Autodesk Inventor part; units mm, degrees
ref_plane "YZ Plane" through (0, 0, 0) normal (1, 0, 0) x (0, 1, 0)
ref_plane "XZ Plane" through (0, 0, 0) normal (0, 1, 0) x (-1, 0, 0)
ref_plane "XY Plane" through (0, 0, 0) normal (0, 0, 1) x (1, 0, 0)
sketch "Sketch1" plane through (0, 0, 0) normal (0, 0, 1) x (1, 0, 0)
  line L0 (0, 0) -> (850.9, 0)
  line L1 (850.9, 0) -> (850.9, 76.2)
  line L2 (850.9, 76.2) -> (0, 76.2)
  line L3 (0, 76.2) -> (0, 0)
  dimension "d0" = 850.9
  dimension "d1" = 76.2
extrude "Extrusion1" add sketch "Sketch1" along normal blind 3.175
sketch "Sketch4" plane through (0, 0, 3.175) normal (0, 0, 1) x (1, 0, 0)
  line L0 (0, 0) -> (0, 38.1)
  line L1 (0, 76.2) -> (0, 0)
  line L2 (0, 0) -> (25.4, 0)
  line L3 (0, 0) -> (850.9, 0)
  line L4 (25.4, 0) -> (0, 38.1)
  line L5 (850.9, 0) -> (825.5, 0)
  line L6 (850.9, 0) -> (850.9, 38.1)
  line L7 (850.9, 0) -> (850.9, 76.2)
  line L8 (850.9, 38.1) -> (825.5, 0)
  line L9 (0, 38.1) -> (0, 36.5125)
  circle A0 centre (292.9509, 36.5125) radius 14.2875
  circle A1 centre (557.9491, 36.5125) radius 14.2875
  circle A2 centre (757.9743, 39.6875) radius 14.2875
  circle A3 centre (92.9257, 39.6875) radius 14.2875
  dimension "d24" = 38.1
  dimension "d26" = 25.4
  dimension "d27" = 38.1
  dimension "d33" = 28.575
  dimension "d34" = 28.575
  dimension "d38" = 28.575
  dimension "d39" = 28.575
extrude "Extrusion3" cut sketch "Sketch4" against normal blind 3.175
sketch "Sketch5" plane through (0, 0, 3.175) normal (0, 0, 1) x (1, 0, 0)
  line L0 (850.9, 76.2) -> (0, 76.2)
  line L1 (0, 76.2) -> (425.45, 76.2)
  circle A0 centre (425.45, 66.675) radius 3.5687
  circle A1 centre (425.45, 9.525) radius 3.5687
  line L2 (25.4, 0) -> (825.5, 0)
  line L3 (0, 76.2) -> (190.5, 76.2)
  circle A2 centre (190.5, 66.675) radius 3.5687
  circle A3 centre (190.5, 9.525) radius 3.5687
  circle A4 centre (190.5, 38.1) radius 3.5687
  line L4 (850.9, 38.1) -> (850.9, 76.2)
  line L5 (850.9, 76.2) -> (660.4, 76.2)
  circle A5 centre (660.4, 66.675) radius 3.5687
  circle A6 centre (660.4, 9.525) radius 3.5687
  circle A7 centre (660.4, 38.1) radius 3.5687
  circle A8 centre (838.2, 63.5) radius 3.5687
  circle A9 centre (12.7, 63.5) radius 3.5687
  line L6 (0, 76.2) -> (0, 38.1)
  circle A10 centre (34.925, 12.7) radius 3.5687
  circle A11 centre (815.975, 12.7) radius 3.5687
  point P0 (0, 0)
  dimension "d42" = 425.45
  dimension "d43" = 7.1374
  dimension "d44" = 9.525
  dimension "d45" = 7.1374
  dimension "d46" = 9.525
  dimension "d47" = 190.5
  dimension "d48" = 7.1374
  dimension "d49" = 9.525
  dimension "d50" = 7.1374
  dimension "d51" = 9.525
  dimension "d52" = 7.1374
  dimension "d53" = 38.1
  dimension "d54" = 190.5
  dimension "d55" = 7.1374
  dimension "d56" = 9.525
  dimension "d57" = 7.1374
  dimension "d58" = 9.525
  dimension "d59" = 7.1374
  dimension "d60" = 38.1
  dimension "d61" = 7.1374
  dimension "d62" = 12.7
  dimension "d63" = 12.7
  dimension "d64" = 7.1374
  dimension "d65" = 12.7
  dimension "d66" = 12.7
  dimension "d67" = 7.1374
  dimension "d69" = 12.7
  dimension "d70" = 9.525
  dimension "d71" = 7.1374
  dimension "d72" = 12.7
  dimension "d73" = 9.525
extrude "Extrusion4" cut sketch "Sketch5" against normal blind 3.175
sketch "Sketch6" plane through (0, 0, 3.175) normal (0, 0, 1) x (1, 0, 0)
  circle A0 centre (190.5, 38.1) radius 3.5687
  circle A1 centre (660.4, 38.1) radius 3.5687
  line L0 (177.673, 25.273) -> (203.327, 25.273)
  line L1 (203.327, 25.273) -> (203.327, 50.927)
  line L2 (203.327, 50.927) -> (177.673, 50.927)
  line L3 (177.673, 50.927) -> (177.673, 25.273)
  line L4 (177.673, 25.273) -> (203.327, 50.927) construction
  line L5 (203.327, 25.273) -> (177.673, 50.927) construction
  line L6 (647.573, 25.273) -> (673.227, 25.273)
  line L7 (673.227, 25.273) -> (673.227, 50.927)
  line L8 (673.227, 50.927) -> (647.573, 50.927)
  line L9 (647.573, 50.927) -> (647.573, 25.273)
  line L10 (647.573, 25.273) -> (673.227, 50.927) construction
  line L11 (673.227, 25.273) -> (647.573, 50.927) construction
  point P0 (0, 0)
  dimension "d76" = 25.654
  dimension "d77" = 25.654
  dimension "d78" = 25.654
  dimension "d79" = 25.654
extrude "Extrusion5" cut sketch "Sketch6" against normal blind 3.175
fillet "Fillet1" radius 1.5875 8 edges at (177.673, 25.273, 1.5875) (203.327, 25.273, 1.5875) (203.327, 50.927, 1.5875) (177.673, 50.927, 1.5875) (647.573, 50.927, 1.5875) (647.573, 25.273, 1.5875) (673.227, 50.927, 1.5875) (673.227, 25.273, 1.5875)
sketch "Sketch7" plane through (0, 0, 3.175) normal (0, 0, 1) x (1, 0, 0)
  circle A0 centre (557.9491, 36.5125) radius 14.2875
  circle A1 centre (534.1366, 36.5125) radius 2.8067
  circle A2 centre (581.7616, 36.5125) radius 2.8067
  circle A3 centre (615.0991, 36.5125) radius 2.8067
  circle A4 centre (499.8313, 36.5125) radius 2.8067
  point P0 (0, 0)
  dimension "d85" = 5.6134
  dimension "d86" = 5.6134
  dimension "d87" = 5.6134
  dimension "d88" = 5.6134
extrude "Extrusion6" cut sketch "Sketch7" against normal blind 25.4 contours A1 | A2 | A3 | A4
sketch "Sketch8" plane through (0, 0, 3.175) normal (0, 0, 1) x (1, 0, 0)
  circle A0 centre (361.95, 38.1) radius 3.5687
  line L0 (850.9, 76.2) -> (0, 76.2)
  line L1 (0, 76.2) -> (0, 38.1)
  circle A1 centre (469.9, 38.1) radius 3.5687
  line L2 (850.9, 38.1) -> (850.9, 76.2)
  point P0 (0, 0)
  dimension "d91" = 7.1374
  dimension "d92" = 38.1
  dimension "d93" = 361.95
  dimension "d94" = 7.1374
  dimension "d95" = 38.1
  dimension "d102" = 381
extrude "Extrusion10" cut sketch "Sketch8" against normal blind 25.4
sketch "Sketch9" plane through (0, 76.2, 0) normal (0, 1, 0) x (1, 0, 0)
  line L0 (850.9, 0) -> (0, 0)
  line L1 (0, 0) -> (0, -3.175)
  line L2 (850.9, -3.175) -> (0, -3.175)
  line L3 (850.9, 0) -> (850.9, -3.175)
extrude "Extrusion11" add sketch "Sketch9" along normal blind 25.4
sketch "Sketch10" plane through (0, 0, 3.175) normal (0, 0, 1) x (1, 0, 0)
  circle A0 centre (12.7, 63.5) radius 3.5687
  circle A1 centre (838.2, 63.5) radius 3.5687
  circle A2 centre (425.45, 66.675) radius 3.5687
  point P0 (0, 0)
extrude "Extrusion13" add sketch "Sketch10" against normal blind 3.175
sketch "Sketch12" plane through (0, 0, 3.175) normal (0, 0, 1) x (1, 0, 0)
  circle A0 centre (12.7, 88.9) radius 3.5687
  circle A1 centre (425.45, 88.9) radius 3.5687
  circle A2 centre (838.2, 88.9) radius 3.5687
  line L0 (850.9, 38.1) -> (850.9, 101.6)
  line L1 (0, 101.6) -> (850.9, 101.6)
  line L2 (0, 38.1) -> (0, 101.6)
  point P0 (0, 0)
  dimension "d113" = 7.1374
  dimension "d114" = 7.1374
  dimension "d115" = 7.1374
  dimension "d116" = 12.7
  dimension "d117" = 12.7
  dimension "d118" = 12.7
  dimension "d119" = 425.45
  dimension "d120" = 12.7
  dimension "d121" = 12.7
extrude "Extrusion14" cut sketch "Sketch12" against normal blind 3.175
sketch "Sketch14" plane through (0, 0, 3.175) normal (0, 0, 1) x (1, 0, 0)
  circle A0 centre (499.8313, 36.5125) radius 2.8067
  point P0 (0, 0)
extrude "Extrusion16" add sketch "Sketch14" against normal blind 3.175
sketch "Sketch15" plane through (0, 0, 3.175) normal (0, 0, 1) x (1, 0, 0)
  circle A0 centre (557.9491, 36.5125) radius 14.2875
  circle A1 centre (500.7991, 36.5125) radius 2.8067
  point P0 (0, 0)
  dimension "d137" = 5.6134
extrude "Extrusion17" cut sketch "Sketch15" against normal blind 3.175 contours A1
sketch "Sketch16" plane through (0, 0, 3.175) normal (0, 0, 1) x (1, 0, 0)
  circle A0 centre (519.9253, 94.3737) radius 4.445
  circle A1 centre (595.9729, 94.3737) radius 4.445
  circle A2 centre (615.0991, 36.5125) radius 2.8067
  circle A3 centre (500.7991, 36.5125) radius 2.8067
  point P0 (0, 0)
  dimension "d140" = 8.89
  dimension "d141" = 8.89
  dimension "d142" = 57.8612
  dimension "d143" = 19.1262
  dimension "d144" = 57.8612
  dimension "d145" = 19.1262
extrude "Extrusion18" cut sketch "Sketch16" against normal blind 3.175 contours A0 | A1
properties part number "InsidePlate2" material "Aluminum 6061"
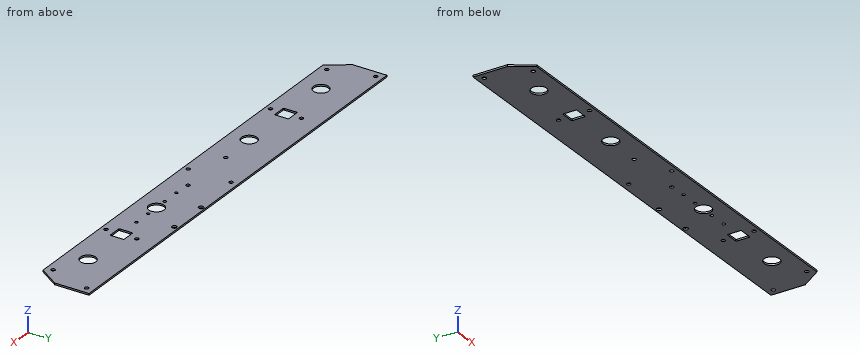
Input: part model. Units: mm. Frame: model coordinates. Round coordinates to 2 decimals unless told otherwise and drop trailing zeros. Loops run counter-clockwise (first coordinate to the right, second up) from the corner with the lowest first, then second, coordinate; pieces in that order, holes last. Notation, with made-up numbers: M -23,-3 L -18,-3 A25 ccw -18,17 Z; hole C 46.25,74 d9. An arc over 180 degrees is marked long. Answer in a Markdown table with one row per item. Add a question column.
1. Section B-B (z = 0.5). Give the number of separate pieces and of enclosed holes in the cut face, and give its area (3 significant figures).
2. Section A-A (x = 551.5). Output: boundary loops of the cut face in (y, z) (3 decimals), and give its area (3 significant figures).
3. Ray query, probe 1 along Y at (x, z) = (190.5, 1.2); probe 2 along X at (y, z) = (89, 2.1); probe 3 along X at (y, z) = (66, 2.1). Return the intervals inside material, ascending.
Values follow:
| question | item | result |
|---|---|---|
| 1 | separate pieces | 1 |
| 1 | enclosed holes | 24 |
| 1 | area | 80,900 mm^2 |
| 2 | outline | M 0,0 L 23.763,0 L 23.763,3.175 L 0,3.175 Z; M 49.262,0 L 101.6,0 L 101.6,3.175 L 49.262,3.175 Z |
| 2 | area | 242 mm^2 |
| 3 | probe 1 | 0 to 5.96, 13.09 to 25.27, 50.93 to 63.11, 70.24 to 101.6 |
| 3 | probe 2 | 0 to 9.13, 16.27 to 421.88, 429.02 to 834.63, 841.77 to 850.9 |
| 3 | probe 3 | 0 to 187, 194 to 656.9, 663.9 to 850.9 |
